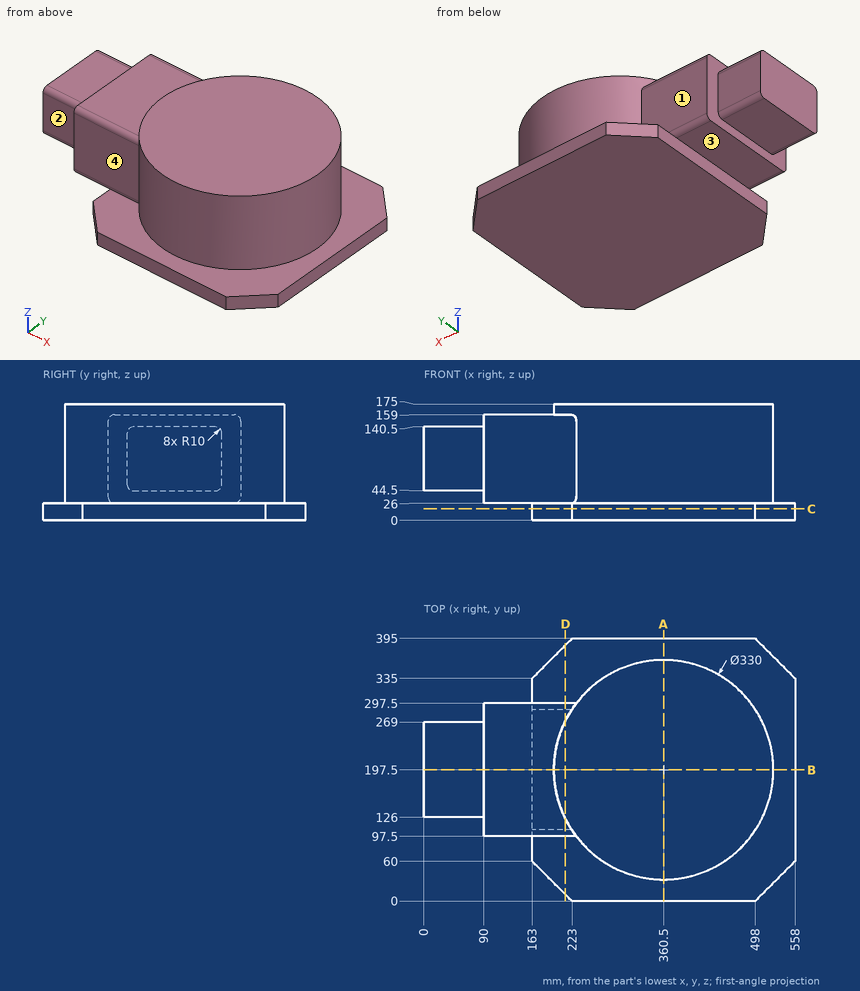
Geometry: see drawing. Coordinates: mm, zero at the bounding-box minimum. A direction names the side the tool comes from. Coordinates: 2 decimals unless noted, no trailing zeros. Loops run counter-clockwise (first coordinate to the right, second up) from the corner with the lowest first, then second, coordinate; pieces in that order, holes last. Notation, with made-up numbers: (73, 73) - (120, 73) arc R25 cw to (120, 112) - close; hole circle Ø9 at (52, -38.75). An arc over 180 degrees is marked (long way). Return JSON: item names as keys, results as strings.
Q1. Material intervals for line 1 along Y through (x, z) = (95, 75.5); line 2 along X through (y, z) = (197, 21); line 3 along Z through (x, y) = (360.5, 19), sorted ascending.
Results:
{"line 1": "97.5 to 297.5", "line 2": "163 to 558", "line 3": "0 to 26"}
Q2. Section A-A, the plane x = 360.5. Return loops of the section in (y, z).
Results:
{"outline": "(0, 0) - (395, 0) - (395, 26) - (362.5, 26) - (362.5, 175) - (32.5, 175) - (32.5, 26) - (0, 26) - close"}
Q3. Contact query for flat-ended pins moving along their axis: P1, Ø5, axis at x = 97.5, z = 129, coming from the +Y side; P2, Ø21, axis at y = 199.5, z = 19.5, coming from the -X side; P3, Ø2, axis at y = 329.5, z = 85, coming from the -X side. Output: stop coordinate, or through.
Results:
{"P1": "y = 297.5", "P2": "x = 90", "P3": "x = 260.18"}
Q4. Access query for the marked faces 1, 2, 3 and 4. Directions: +Z, -Z, +X, -X, +Y, -Y. A direction counts if a zero-diameter tool reaches every point of the face in a straight line with its end or side. Return the directions, or none.
Results:
{"face 1": "+Z, -X, +Y", "face 2": "+Z, -Z, -X, -Y", "face 3": "-Z, -X, +Y, -Y", "face 4": "+Z, -X, -Y"}
Q5. Section C-C, the plane z = 17.5. Return loops of the section in (x, y), plus the area to 3 significant figures.
Results:
{"outline": "(163, 60) - (223, 0) - (498, 0) - (558, 60) - (558, 335) - (498, 395) - (223, 395) - (163, 335) - close", "area": "149,000 mm2"}
Q6. Section D-D, the plane x = 213. Return loops of the section in (y, z).
Results:
{"outline": "(10, 0) - (385, 0) - (385, 26) - (287.5, 26) arc R10 ccw to (297.5, 36) - (297.5, 149) arc R10 ccw to (287.5, 159) - (271.45, 159) - (271.45, 175) - (123.55, 175) - (123.55, 159) - (107.5, 159) arc R10 ccw to (97.5, 149) - (97.5, 36) arc R10 ccw to (107.5, 26) - (10, 26) - close"}
Q7. Section B-B, the plane y = 197.5. Return loops of the section in (x, z).
Results:
{"outline": "(0, 44.5) - (90, 44.5) - (90, 26) - (163, 26) - (163, 0) - (558, 0) - (558, 26) - (525.5, 26) - (525.5, 175) - (195.5, 175) - (195.5, 159) - (90, 159) - (90, 140.5) - (0, 140.5) - close"}
